Work out the finished part from the listing and answer in its coordinate system (mm). Round coordinates to 2 decimals unless told otherwise and drop trailing zeros. Write each loop counter-clockwise with the first axis right and the second up, starting at its lowest first coordinate (ties: lowest second). Pieces come first, ordered by that corner, then holes. Notation, with made-up numbers: (6.25, -37.5) - (14.25, -37.5) arc R17 cw to (14.25, -19.5) - close; hole circle Ø11 at (-36.5, 67). An arc over 180 degrees is marked (long way). Answer as a JSON object with one key per item and string values.
Autodesk Inventor part; units mm, degrees
ref_plane "YZ Plane" through (0, 0, 0) normal (1, 0, 0) x (0, 1, 0)
ref_plane "XZ Plane" through (0, 0, 0) normal (0, 1, 0) x (-1, 0, 0)
ref_plane "XY Plane" through (0, 0, 0) normal (0, 0, 1) x (1, 0, 0)
sketch "Эскиз1" plane through (0, 0, 0) normal (0, 1, 0) x (-1, 0, 0)
  line L0 (-200, 65) -> (200, 65) construction
  line L1 (200, 65) -> (200, -65) construction
  line L2 (200, -65) -> (-200, -65) construction
  line L3 (-200, -65) -> (-200, 65) construction
  line L4 (-200, 65) -> (200, -65) construction
  line L5 (200, 65) -> (-200, -65) construction
  line L6 (200, 65) -> (180, 65)
  line L7 (180, 65) -> (180, 45)
  line L8 (180, 45) -> (200, 45)
  line L9 (200, 45) -> (200, 65)
  line L10 (200, -65) -> (180, -65)
  line L11 (180, -65) -> (180, -45)
  line L12 (180, -45) -> (200, -45)
  line L13 (200, -45) -> (200, -65)
  line L14 (-200, 65) -> (-180, 65)
  line L15 (-180, 65) -> (-180, 45)
  line L16 (-180, 45) -> (-200, 45)
  line L17 (-200, 45) -> (-200, 65)
  line L18 (-200, -65) -> (-180, -65)
  line L19 (-180, -65) -> (-180, -45)
  line L20 (-180, -45) -> (-200, -45)
  line L21 (-200, -45) -> (-200, -65)
  point P0 (0, 0)
  dimension "d0" = 400
  dimension "d1" = 130
  dimension "d2" = 20
  dimension "d3" = 20
  dimension "d4" = 20
  dimension "d5" = 20
  dimension "d6" = 20
  dimension "d7" = 20
  dimension "d8" = 20
  dimension "d9" = 20
extrude "Выдавливание1" add sketch "Эскиз1" along normal blind 400
sketch "Эскиз2" plane through (200, 0, 65) normal (1, 0, 0) x (0, 0, -1)
  line L0 (20, 400) -> (0, 400)
  line L1 (0, 400) -> (20, 400)
  line L2 (20, 400) -> (20, 420)
  line L3 (20, 420) -> (0, 420)
  line L4 (0, 420) -> (0, 400)
  line L5 (130, 0) -> (130, 400)
  line L6 (130, 400) -> (110, 400)
  line L7 (110, 400) -> (110, 420)
  line L8 (110, 420) -> (130, 420)
  line L9 (130, 420) -> (130, 400)
  line L10 (0, 0) -> (0, 400)
  line L11 (0, 280) -> (20, 280)
  line L12 (20, 280) -> (20, 300)
  line L13 (20, 300) -> (0, 300)
  line L14 (0, 300) -> (0, 280)
  line L15 (110, 300) -> (130, 300)
  line L16 (130, 300) -> (130, 280)
  line L17 (130, 280) -> (110, 280)
  line L18 (110, 280) -> (110, 300)
  point P0 (65, 0)
  point P1 (0, 300)
  dimension "d12" = 20
  dimension "d13" = 20
  dimension "d14" = 20
  dimension "d15" = 20
  dimension "d25" = 20
  dimension "d26" = 20
  dimension "d27" = 100
  dimension "d28" = 20
  dimension "d29" = 20
  dimension "d30" = 100
  dimension "d31" = 90
extrude "Выдавливание2" add sketch "Эскиз2" against normal blind 400
sketch "Эскиз3" plane through (-200, 420, 65) normal (0, 0, 1) x (1, 0, 0)
  line L0 (0, -420) -> (0, 0)
  line L1 (20, -420) -> (20, -20)
  line L2 (0, 0) -> (20, 0)
  line L3 (20, 0) -> (20, -20)
  line L4 (20, -20) -> (0, -20)
  line L5 (0, -20) -> (0, 0)
  line L6 (380, -420) -> (380, -20)
  line L7 (400, -420) -> (400, 0)
  line L8 (380, -20) -> (400, -20)
  line L9 (400, -20) -> (400, 0)
  line L10 (400, 0) -> (380, 0)
  line L11 (380, 0) -> (380, -20)
  line L12 (0, -140) -> (20, -140)
  line L13 (20, -140) -> (20, -120)
  line L14 (20, -120) -> (0, -120)
  line L15 (0, -120) -> (0, -140)
  line L16 (380, -420) -> (380, -20)
  line L17 (400, -420) -> (400, 0)
  line L18 (380, -140) -> (400, -140)
  line L19 (400, -140) -> (400, -120)
  line L20 (400, -120) -> (380, -120)
  line L21 (380, -120) -> (380, -140)
  point P0 (200, -420)
  point P1 (20, -120)
  point P2 (0, -120)
  point P3 (20, -140)
  dimension "d20" = 20
  dimension "d21" = 20
  dimension "d22" = 100
  dimension "d23" = 100
  dimension "d24" = 20
extrude "Выдавливание3" add sketch "Эскиз3" against normal blind 130 contours L0 L14 L1 L12 | L0 L2 L3 L4 | L6 L20 L7 L18 | L11 L10 L7 L8
sketch "Эскиз4" plane through (200, 420, -65) normal (0, 0, -1) x (-1, 0, 0)
  point P0 (200, -420)
sketch "Эскиз7" plane through (0, 0, 0) normal (0, -1, 0) x (1, 0, 0)
  line L0 (232.9472, 106.3053) -> (134.9615, 106.3053)
  line L1 (134.9615, 106.3053) -> (134.9615, -101.9914)
  line L2 (134.9615, -101.9914) -> (232.9472, -101.9914)
  line L3 (232.9472, -101.9914) -> (232.9472, 106.3053)
  point P0 (0, 0)
extrude "Выдавливание5" cut sketch "Эскиз7" against normal blind 80
sketch "Эскиз9" plane through (0, 0, 0) normal (0, 0, 1) x (1, 0, 0)
  line L0 (200, 80) -> (180, 80)
  line L1 (200, 80) -> (180, 80)
  line L2 (180, 80) -> (180, 60)
  line L3 (180, 60) -> (200, 60)
  line L4 (200, 60) -> (200, 80)
  point P0 (0, 0)
  dimension "d45" = 20
  dimension "d46" = 20
extrude "Выдавливание6" add sketch "Эскиз9" along normal mid plane 130
sketch "Эскиз11" plane through (180, 60, 65) normal (0, -1, 0) x (1, 0, 0)
  line L0 (0, -20) -> (20, -20)
  line L1 (20, -110) -> (0, -110)
  point P0 (-180, -65)
  point P1 (10, -20)
  point P2 (10, -110)
hole "Отверстие3" at (190, 60, 45) at (190, 60, -45) direction (0, 1, 0) diameter 5 depth 5
properties part number "Подлокотник"
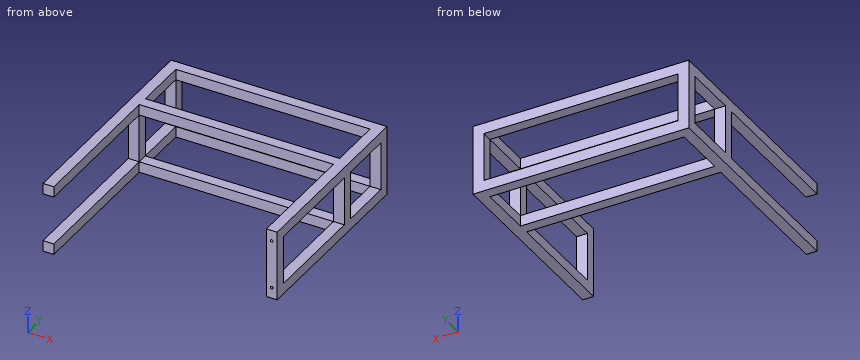
Item 1: Each of these flat-tipped pins is pushed along its axis until it touches: P1, Ø10, axis at x = -191, z = -16, coming from the -Y side; P2, Ø10, axis at x = 193, z = 22.5, coming from the -Y side. Where does it stop, or does it pass through?
Results found:
{"P1": "y = 280", "P2": "y = 60"}
Item 2: A cutting plane is placed at C-C (z = 20.5). Write down the section's boundary in (x, y).
Results found:
{"outline": "(-200, 280) - (-180, 280) - (-180, 300) - (-200, 300) - close; (-200, 400) - (-180, 400) - (-180, 420) - (-200, 420) - close; (180, 60) - (200, 60) - (200, 80) - (180, 80) - close; (180, 280) - (200, 280) - (200, 300) - (180, 300) - close; (180, 400) - (200, 400) - (200, 420) - (180, 420) - close"}
Item 3: A cutting plane is placed at A-A (y = 161.5). Write down the section's boundary in (x, z), and give its area (3 significant figures).
Results found:
{"outline": "(-200, -65) - (-180, -65) - (-180, -45) - (-200, -45) - close; (-200, 45) - (-180, 45) - (-180, 65) - (-200, 65) - close; (180, -65) - (200, -65) - (200, -45) - (180, -45) - close; (180, 45) - (200, 45) - (200, 65) - (180, 65) - close", "area": "1,600 mm²"}
Item 4: A cutting plane is placed at D-D (x = -18). Write down the section's boundary in (y, z).
Results found:
{"outline": "(280, -65) - (300, -65) - (300, -45) - (280, -45) - close; (280, 45) - (300, 45) - (300, 65) - (280, 65) - close; (400, -65) - (420, -65) - (420, -45) - (400, -45) - close; (400, 45) - (420, 45) - (420, 65) - (400, 65) - close"}
Item 5: Consider line 1 along Z through (x, y) = (190, 63); line 2 along X through (y, z) = (357.5, 59.5); line 3 along Y through (x, z) = (-13, -53). Determine where each line is inside the solid, lowest interval first.
Results found:
{"line 1": "-65 to -47.5, -42.5 to 42.5, 47.5 to 65", "line 2": "-200 to -180, 180 to 200", "line 3": "280 to 300, 400 to 420"}
Item 6: A cutting plane is placed at B-B (y = 42.5). Write down the section's boundary in (x, z), and give its area (3 significant figures).
Results found:
{"outline": "(-200, -65) - (-180, -65) - (-180, -45) - (-200, -45) - close; (-200, 45) - (-180, 45) - (-180, 65) - (-200, 65) - close", "area": "800 mm²"}
